Answer from the drawing. Dimensions are ordinates in mm from the lowest x, y and z of the part. A direction names the side the tool comes from. Coordinates: 2 decimals unless noted, no trailing zeros. Loops run counter-clockwise (first coordinate to the right, second up) from the corner with the lowest first, then second, coordinate; pieces in that order, holes last.
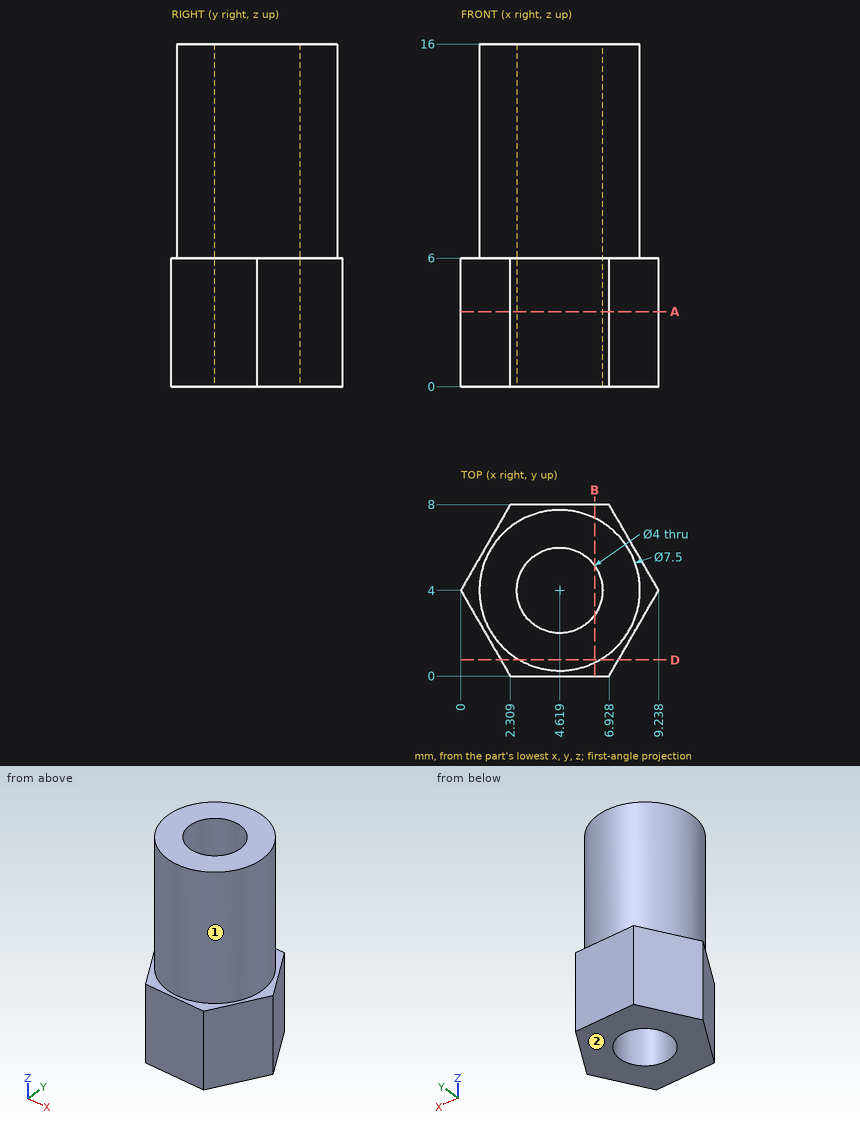
Item 1: A cutting plane is placed at D-D on y = 0.75. Determine the outline of the cut face in (x, z).
Numbers:
outline: (1.88, 0) - (7.36, 0) - (7.36, 6) - (6.49, 6) - (6.49, 16) - (2.75, 16) - (2.75, 6) - (1.88, 6) - close
Item 2: Find the intervals of material crossed by line 1 along Y through (x, z) = (4.5, 8); line 2 along X through (y, z) = (5, 4.5); line 3 along Y through (x, z) = (5, 2.25), in increasing order.
Numbers:
line 1: y = 0.25 to 2, 6 to 7.75
line 2: x = 0.58 to 2.89, 6.35 to 8.66
line 3: y = 0 to 2.04, 5.96 to 8
Item 3: Given pin 1 (2 mm diameter, centred on x = 3.5, z = 8, fed in from +Y); pin 2 (4 mm diameter, centred on y = 6.5, z = 10, fed in from +X) (1 decimal), each flat-ended and moving along its own axis, determine where each tip first touches the part or whether it passes through.
Numbers:
pin 1: stops at y = 7.75
pin 2: stops at x = 8.3
Item 4: Which of the six approach directions +Z, -Z, +X, -X, +Y, -Y give full straight-line access (tool end or side, diameter ignored) to the marked faces 1 and 2?
Numbers:
face 1: +Z
face 2: -Z, +X, -X, +Y, -Y
Item 5: A cutting plane is placed at A-A on z = 3.5. Determine the outline of the cut face in (x, y).
Numbers:
outline: (0, 4) - (2.31, 0) - (6.93, 0) - (9.24, 4) - (6.93, 8) - (2.31, 8) - close; hole circle Ø4 at (4.62, 4)
Item 6: A cutting plane is placed at B-B on x = 6.25. Determine the outline of the cut face in (y, z).
Numbers:
outline: (0, 0) - (2.84, 0) - (2.84, 16) - (0.62, 16) - (0.62, 6) - (0, 6) - close; (5.16, 0) - (8, 0) - (8, 6) - (7.38, 6) - (7.38, 16) - (5.16, 16) - close
